Can you work these out from the model? Positions are in its coordinate system, mm. Round coordinates to 2 decimals unless told otherwise and drop trailing zeros. Order: outer loops, then holes, each group sorted by start corner. A loop starts at its lowest first (then second) coordinate and runs counter-clockwise, first axis right, second up. Notation, with made-up numbers: M 80.25,71 L 119.25,71 A30 cw 119.25,98 Z; hole C 69.25,39.5 d10. An arc over 180 degrees is marked long. Answer as a JSON object with one key per item and string values. Group by question number.
```python
from build123d import *

# Parameters (mm, degrees)
SKETCH_W     = 31.83
SKETCH_H     = 31.24
PAD_DEPTH    = 1.5
FILLET_R     = 1
POCKET_DEPTH = 0.9
SKETCH028_W  = 28
SKETCH028_H  = 27
PAD021_DEPTH = 0.8


with BuildPart() as part:
    # Sketch → Pad (new body)
    with BuildSketch(Plane(origin=(0, 0, 0), x_dir=(-1, 0, 0), z_dir=(0, 0, -1))):
        with Locations((-16.895, 25.69)):
            Rectangle(SKETCH_W, SKETCH_H)
    extrude(amount=PAD_DEPTH)

    # Fillet
    fillet_edges = [part.edges().sort_by_distance(p)[0] for p in [
        (32.81, 41.31, -0.75),
        (0.98, 41.31, -0.75),
        (0.98, 10.07, -0.75),
        (32.81, 10.07, -0.75),
    ]]
    fillet(fillet_edges, radius=FILLET_R)

    # Fillet Face2 → Pocket (cut)
    with BuildSketch(Plane(origin=(16.895, 25.69, 0), x_dir=(0, 1, 0), z_dir=(0, 0, 1))):
        with BuildLine():
            Line((15.62, -14.915), (15.62, 14.915))
            ThreePointArc((15.62, 14.915), (15.327107, 15.622107), (14.62, 15.915))
            Line((14.62, 15.915), (-14.62, 15.915))
            ThreePointArc((-14.62, 15.915), (-15.327107, 15.622107), (-15.62, 14.915))
            Line((-15.62, 14.915), (-15.62, -14.915))
            ThreePointArc((-15.62, -14.915), (-15.327107, -15.622107), (-14.62, -15.915))
            Line((-14.62, -15.915), (14.62, -15.915))
            ThreePointArc((14.62, -15.915), (15.327107, -15.622107), (15.62, -14.915))
        make_face()
    extrude(amount=-POCKET_DEPTH, mode=Mode.SUBTRACT)

    # Sketch028 (on Face4 of Pocket) → Pad021 (join)
    with BuildSketch(Plane(origin=(0, 0, -1.5), x_dir=(1, 0, 0), z_dir=(0, 0, -1))):
        with Locations((17, -25.8)):
            Rectangle(SKETCH028_W, SKETCH028_H)
    extrude(amount=PAD021_DEPTH)


solid = part.part
```
1) If we section it at B-B on x = 6: Write out the boundary of the cut face in (y, z).
2) If we section it at C-C on z = -1.95: Write out the boundary of the cut face in (x, y), plus the area to 3 significant figures.
3) If we section it at A-A on y = 25.5: Write out the boundary of the cut face in (x, z), plus the area to 3 significant figures.
4) I need wall thicknesses on line 1 along Z through (x, y) = (21.5, 40.5); line 2 along X through (y, z) = (22, -1.9); line 3 along Y through (x, z) = (12, -1.9). Which ranges of each line are inside material? Lowest first, please.
Findings:
{
 "1": {"outline": "M 10.07,-1.5 L 12.3,-1.5 L 12.3,-2.3 L 39.3,-2.3 L 39.3,-1.5 L 41.31,-1.5 L 41.31,-0.9 L 10.07,-0.9 Z"},
 "2": {"outline": "M 3,12.3 L 31,12.3 L 31,39.3 L 3,39.3 Z", "area": "756 mm^2"},
 "3": {"outline": "M 0.98,-1.5 L 3,-1.5 L 3,-2.3 L 31,-2.3 L 31,-1.5 L 32.81,-1.5 L 32.81,-0.9 L 0.98,-0.9 Z", "area": "41.5 mm^2"},
 "4": {"line 1": "z = -1.5 to -0.9", "line 2": "x = 3 to 31", "line 3": "y = 12.3 to 39.3"}
}
